Build history of the part. All positions in model axes, mm. A direction names the side the tool comes from. Give positions to 0.01 mm unless a question says otherwise; leave off trailing zeros. Loops run counter-clockwise (first coordinate to the right, second up) from the corner with the lowest first, then second, coordinate; pieces in that order, holes last. Notation, with made-up numbers: (12, 3) - (31, 3) arc R21 cw to (31, 16) - close; hole circle Ø1 at (33.5, 3.5). An arc over 180 degrees is marked (long way). Return JSON: item names as keys, results as strings. Group by question number.
1) Slice it at C-C (x = 25.4). List the corners of the cut face in (y, z), and give its area (3 significant figures).
2) Mould opens along Z. For faces 4 (the face through (56, 9, 0)), 5 (the face through (6.35, 9, -39)), 6 (the face through (99.225, 6, -51)) say: released by +Z, released by -Z, zero draft, split by the parting line, or undercut.
3) Drop a flat-ended pin along its axis: pin 1 (10.5 mm diameter, centred on x = 85.5, z = -61, fed in from -Y). Give the stop position or say it passes through.
4) 3-axis set-ups, long thin cutter, end or side, ignore diameter. For faces 1 (the face through (78.575, 6, -51)), 2 (the face through (89.06, 15.83, -30.99)), 3 (the face through (56, 19.05, -39)): which of +Z, -Z, +X, -X, +Y, -Y reach the whole face in a straight line?
5) Slice it at D-D (y = 17). List the corners of the cut face in (x, z).
6) Drill centre lines: probe 1 along Z at (x, y) = (88.9, 14.25); probe 2 along Z at (x, y) = (88.9, 9.5); probe 3 along X at (y, z) = (16.25, -40.5). Where is each one in solid material? Low to high. Write a range as from..to.
7) Slice it at A-A (y = 3.5). List the corners of the cut face in (x, z), and give its area (3 significant figures).
8) Slice it at B-B (z = -45). List the corners of the cut face in (x, y), and give its area (3 significant figures).
```python
from build123d import *

# Parameters (mm, degrees)
SKETCH1_W               = 114.3
SKETCH1_H               = 76.2
BASE_EXTRUDE_DEPTH      = 19.05
F_1_2_20_TAPPED_HOLE1_D = 12.7
CUT_EXTRUDE1_DEPTH      = 12.7
CUT_EXTRUDE2_DEPTH      = 12.7
SKETCH7_W               = 6.35
SKETCH7_H               = 76.2
CUT_EXTRUDE3_DEPTH      = 1
CUT_EXTRUDE3_DEPTH_BACK = 20.05
SKETCH8_W               = 6.35
SKETCH8_H               = 76.2
CUT_EXTRUDE4_DEPTH      = 1
CUT_EXTRUDE4_DEPTH_BACK = 20.05


with BuildPart() as part:
    # Sketch1 → Base-Extrude (new body)
    with BuildSketch(Plane(origin=(0, 0, 0), x_dir=(1, 0, 0), z_dir=(0, 1, 0))):
        with Locations((57.15, 38.1)):
            Rectangle(SKETCH1_W, SKETCH1_H)
        with BuildLine():
            Line((96.012, 63.5), (96.012, 38.1))
            ThreePointArc((96.012, 38.1), (88.9, 30.988), (81.788, 38.1))
            Line((81.788, 38.1), (81.788, 63.5))
            ThreePointArc((81.788, 63.5), (88.9, 70.612), (96.012, 63.5))
        make_face(mode=Mode.SUBTRACT)
        with BuildLine():
            Line((18.288, 63.5), (18.288, 38.1))
            ThreePointArc((18.288, 38.1), (25.4, 30.988), (32.512, 38.1))
            Line((32.512, 38.1), (32.512, 63.5))
            ThreePointArc((32.512, 63.5), (25.4, 70.612), (18.288, 63.5))
        make_face(mode=Mode.SUBTRACT)
    extrude(amount=BASE_EXTRUDE_DEPTH)

    # 1/2-20 Tapped Hole1 (through all)
    with Locations(Plane(origin=(0, 19.05, 0), x_dir=(-1, 0, 0), z_dir=(0, 1, 0))):
        with Locations((-25.4, -19.05), (-88.9, -19.05)):
            Hole(F_1_2_20_TAPPED_HOLE1_D / 2)

    # Sketch4 → Cut-Extrude1 (cut)
    with BuildSketch(Plane.XZ):
        with BuildLine():
            Line((15.0749, -63.5), (15.0749, -38.1))
            ThreePointArc((15.0749, -38.1), (25.4, -27.7749), (35.7251, -38.1))
            Line((35.7251, -38.1), (35.7251, -63.5))
            ThreePointArc((35.7251, -63.5), (25.4, -73.8251), (15.0749, -63.5))
        make_face()
    extrude(amount=-CUT_EXTRUDE1_DEPTH, mode=Mode.SUBTRACT)

    # Sketch5 → Cut-Extrude2 (cut)
    with BuildSketch(Plane.XZ):
        with BuildLine():
            Line((99.2251, -38.1), (99.2251, -63.5))
            ThreePointArc((99.2251, -63.5), (88.9, -73.8251), (78.5749, -63.5))
            Line((78.5749, -63.5), (78.5749, -38.1))
            ThreePointArc((78.5749, -38.1), (88.9, -27.7749), (99.2251, -38.1))
        make_face()
    extrude(amount=-CUT_EXTRUDE2_DEPTH, mode=Mode.SUBTRACT)

    # Sketch7 → Cut-Extrude3 (cut, two sides)
    with BuildSketch(Plane.XZ) as cut_extrude3_sk:
        with Locations((111.125, -38.1)):
            Rectangle(SKETCH7_W, SKETCH7_H)
    extrude(amount=CUT_EXTRUDE3_DEPTH, mode=Mode.SUBTRACT)
    extrude(cut_extrude3_sk.sketch, amount=-CUT_EXTRUDE3_DEPTH_BACK, mode=Mode.SUBTRACT)

    # Sketch8 → Cut-Extrude4 (cut, two sides)
    with BuildSketch(Plane.XZ) as cut_extrude4_sk:
        with Locations((3.175, -38.1)):
            Rectangle(SKETCH8_W, SKETCH8_H)
    extrude(amount=CUT_EXTRUDE4_DEPTH, mode=Mode.SUBTRACT)
    extrude(cut_extrude4_sk.sketch, amount=-CUT_EXTRUDE4_DEPTH_BACK, mode=Mode.SUBTRACT)


solid = part.part
```
Results:
{
 "1": {"outline": "(0, -76.2) - (19.05, -76.2) - (19.05, -70.61) - (12.7, -70.61) - (12.7, -73.83) - (0, -73.83) - close; (0, -27.77) - (12.7, -27.77) - (12.7, -30.99) - (19.05, -30.99) - (19.05, -25.4) - (0, -25.4) - close; (0, -12.7) - (19.05, -12.7) - (19.05, 0) - (0, 0) - close", "area": "373 mm2"},
 "2": {"face 4": "released by +Z", "face 5": "zero draft", "face 6": "undercut"},
 "3": {"pin 1": "y = 12.7"},
 "4": {"face 1": "-Y", "face 2": "+Y, -Y", "face 3": "+Z, -Z, +X, -X, +Y"},
 "5": {"outline": "(6.35, -76.2) - (107.95, -76.2) - (107.95, 0) - (6.35, 0) - close; hole (18.29, -63.5) arc R7.11 ccw to (32.51, -63.5) - (32.51, -38.1) arc R7.11 ccw to (18.29, -38.1) - close; hole circle Ø12.7 at (25.4, -19.05); hole (81.79, -63.5) arc R7.11 ccw to (96.01, -63.5) - (96.01, -38.1) arc R7.11 ccw to (81.79, -38.1) - close; hole circle Ø12.7 at (88.9, -19.05)"},
 "6": {"probe 1": "-76.2..-70.61, -30.99..-25.4, -12.7..0", "probe 2": "-76.2..-73.83, -27.77..-25.4, -12.7..0", "probe 3": "6.35..18.29, 32.51..81.79, 96.01..107.95"},
 "7": {"outline": "(6.35, -76.2) - (107.95, -76.2) - (107.95, 0) - (6.35, 0) - close; hole (15.07, -63.5) arc R10.33 ccw to (35.73, -63.5) - (35.73, -38.1) arc R10.33 ccw to (15.07, -38.1) - close; hole circle Ø12.7 at (25.4, -19.05); hole (78.57, -63.5) arc R10.33 ccw to (99.23, -63.5) - (99.23, -38.1) arc R10.33 ccw to (78.57, -38.1) - close; hole circle Ø12.7 at (88.9, -19.05)", "area": "5,770 mm2"},
 "8": {"outline": "(6.35, 0) - (15.07, 0) - (15.07, 12.7) - (18.29, 12.7) - (18.29, 19.05) - (6.35, 19.05) - close; (32.51, 12.7) - (35.73, 12.7) - (35.73, 0) - (78.57, 0) - (78.57, 12.7) - (81.79, 12.7) - (81.79, 19.05) - (32.51, 19.05) - close; (96.01, 12.7) - (99.23, 12.7) - (99.23, 0) - (107.95, 0) - (107.95, 19.05) - (96.01, 19.05) - close", "area": "1,230 mm2"}
}
